```python
from build123d import *

# Parameters (mm, degrees)
F0_R     = 10.9728
F1_DEPTH = 6.9342


# Not quite as in the source:
# - a feature names something its author has since deleted; it is built from what else it names


with BuildPart() as f1:
    # F0 (on Front) → F1 (new body)
    with BuildSketch(Plane.XZ):
        with BuildLine():
            ThreePointArc((28.6439371533, 44.738406593), (31.7550616118, 42.5865732614), (34.7051660635, 40.2187967078))
            Line((34.7051660635, 40.2187967078), (38.3958422982, 44.2064153225))
            ThreePointArc((38.3958422982, 44.2064153225), (36.1509937048, 46.060324745), (33.8167671779, 47.8003568929))
            Line((33.8167671779, 47.8003568929), (28.6439371533, 44.738406593))
        make_face()
        with BuildLine():
            Line((38.3958422982, 44.2064153225), (34.7051660635, 40.2187967078))
            ThreePointArc((34.7051660635, 40.2187967078), (48.2991997583, 22.1175826623), (53.1225014483, 0))
            ThreePointArc((53.1225014483, 0), (24.8760182095, -46.9380855826), (-29.8247927528, -43.9600033823))
            Line((-29.8247927528, -43.9600033823), (-35.1168298869, -46.8535603786))
            ThreePointArc((-35.1168298869, -46.8535603786), (26.1940251259, -52.3671739658), (58.5529492123, 0))
            ThreePointArc((58.5529492123, 0), (53.2758747723, 24.2925714716), (38.3958422982, 44.2064153225))
        make_face()
        with BuildLine():
            ThreePointArc((33.8167671779, 47.8003568929), (36.1509937048, 46.060324745), (38.3958422982, 44.2064153225))
            Line((38.3958422982, 44.2064153225), (51.3007947444, 58.1496672696))
            Line((51.3007947444, 58.1496672696), (33.8167671779, 47.8003568929))
        make_face()
        with BuildLine():
            ThreePointArc((-37.1603482471, -37.9619372303), (-41.568846888, 33.0761413789), (28.6439371533, 44.738406593))
            Line((28.6439371533, 44.738406593), (33.8167671779, 47.8003568929))
            ThreePointArc((33.8167671779, 47.8003568929), (-44.9890332079, 37.475788884), (-40.9020715179, -41.898310312))
            Line((-40.9020715179, -41.898310312), (-37.1603482471, -37.9619372303))
        make_face()
        with BuildLine():
            Line((-35.1168298869, -46.8535603786), (-29.8247927528, -43.9600033823))
            ThreePointArc((-29.8247927528, -43.9600033823), (-33.6265739867, -41.1248547965), (-37.1603482471, -37.9619372303))
            Line((-37.1603482471, -37.9619372303), (-40.9020715179, -41.898310312))
            ThreePointArc((-40.9020715179, -41.898310312), (-38.090116415, -44.4701123559), (-35.1168298869, -46.8535603786))
        make_face()
        with BuildLine():
            Line((-56.9704473019, -58.8025860488), (-35.1168298869, -46.8535603786))
            ThreePointArc((-35.1168298869, -46.8535603786), (-38.090116415, -44.4701123559), (-40.9020715179, -41.898310312))
            Line((-40.9020715179, -41.898310312), (-56.9704473019, -58.8025860488))
        make_face()
        with BuildLine():
            Line((38.8165365087, 20.8673397533), (16.7947365087, 20.8673397533))
            Line((16.7947365087, 20.8673397533), (34.7051660635, 40.2187967078))
            ThreePointArc((34.7051660635, 40.2187967078), (31.7550616118, 42.5865732614), (28.6439371533, 44.738406593))
            Line((28.6439371533, 44.738406593), (-32.8515800228, 8.3374004968))
            Line((-32.8515800228, 8.3374004968), (-11.6390858311, 8.3374004968))
            Line((-11.6390858311, 8.3374004968), (-43.993112864, -21.982746443))
            Line((-43.993112864, -21.982746443), (-21.971312864, -21.982746443))
            Line((-21.971312864, -21.982746443), (-37.1603482471, -37.9619372303))
            ThreePointArc((-37.1603482471, -37.9619372303), (-33.6265739867, -41.1248547965), (-29.8247927528, -43.9600033823))
            Line((-29.8247927528, -43.9600033823), (31.308234758, -10.5339530787))
            Line((31.308234758, -10.5339530787), (10.099234758, -10.5339530787))
            Line((10.099234758, -10.5339530787), (38.8165365087, 20.8673397533))
        make_face()
        Circle(F0_R, mode=Mode.SUBTRACT)
    extrude(amount=F1_DEPTH)


solid = f1.part
```
CAD build for the part. Positions are in the model's coordinates, mm. A direction names the side the tool comes from. Round coordinates to 2 decimals unless told otherwise and drop trailing zeros. Loops run counter-clockwise (first coordinate to the right, second up) from the corner with the lowest first, then second, coordinate; pieces in that order, holes last. Notation, with made-up numbers: (89, 70.5) - (106, 70.5) arc R34 cw to (106, 107.5) - close; hole circle Ø3 at (36, 20). An arc over 180 degrees is marked (long way). Return JSON: item names as keys, results as strings. Group by question number.
Q1. Band-saw the part on B-B on z = -4.5. Give the cut face in (x, y).
Q2. Tool access for faces 1 (the face through (28, -3, 20.867)), 2 (the face through (42.681, -3.419, 53.047)), 3 (the face through (-46.197, -3.419, -52.912)), 4 (the face through (-1, -6.934, -12)): list every direction of +Z, -Z, +X, -X, +Y, -Y with a clear straight run to the whole face (end or side of a thin tool).
Q3. Drill centre lines: line 1 along Z through (x, y) = (1.5, -3.25); line 2 along Z through (x, y) = (-20, -2); line 3 along Z through (x, y) = (32.5, -5.5). Where is each one in solid material? Low to high. Write a range as [from, to].
Q4. Two-plate mould, pull along X, no slides. Class faces 5 (the face through (-48.82, -3.42, -50.23)), 6 (the face through (-1, 0, -12)), 7 (the face through (44.76, -3.42, 51.08)), 8 (the face through (-1.673, -3.419, 26.793)): +X half, -X half, draft (parallel to the pull), parting line (faces both ways), or undercut.
Q5. Band-saw the part on D-D on z = -40.5. Give the cut face in (x, y).
Q6. Band-saw the part on C-C on x = -15.5. Give the cut face in (y, z), plus the area to 3 significant figures.
Q7. Flat gauge pins, fed straight in: pin 1 Ø12 at (x, z) = (28.5, -21) entering from +Y; pin 2 Ø3 at (x, y) = (18, -4.5) entering from +Z; pin 3 Ø1.5 at (y, z) = (-2.5, -38.5) entering from -X; pin 4 Ø3.5 at (x, y) = (-19.5, -4.5) entering from -Z. Where does each tip first touch, or does it go through?
Solutions:
{
 "1": {"outline": "(-58.38, -6.93) - (-52.93, -6.93) - (-52.93, 0) - (-58.38, 0) - close; (-25.34, -6.93) - (-10.01, -6.93) - (-10.01, 0) - (-25.34, 0) - close; (10.01, -6.93) - (15.62, -6.93) - (15.62, 0) - (10.01, 0) - close; (52.93, -6.93) - (58.38, -6.93) - (58.38, 0) - (52.93, 0) - close"},
 "2": {"face 1": "+Y, -Y", "face 2": "+Z, +Y, -Y", "face 3": "-Z, +Y, -Y", "face 4": "+Z, -Z, +X, -X, -Y"},
 "3": {"line 1": "z = [-58.53, -53.1], [-26.83, -10.87], [10.87, 28.67], [53.1, 58.53]", "line 2": "z = [-55.03, -49.21], [-38.59, 0.5], [8.34, 15.94], [49.21, 55.03]", "line 3": "z = [-48.71, -42.02], [13.96, 20.87], [37.84, 48.71]"},
 "4": {"face 5": "-X half", "face 6": "draft", "face 7": "+X half", "face 8": "undercut"},
 "5": {"outline": "(-42.29, -6.93) - (-23.5, -6.93) - (-23.5, 0) - (-42.29, 0) - close; (34.38, -6.93) - (42.29, -6.93) - (42.29, 0) - (34.38, 0) - close"},
 "6": {"outline": "(-6.93, -56.46) - (0, -56.46) - (0, -50.81) - (-6.93, -50.81) - close; (-6.93, -36.13) - (0, -36.13) - (0, 4.72) - (-6.93, 4.72) - close; (-6.93, 8.34) - (0, 8.34) - (0, 18.61) - (-6.93, 18.61) - close; (-6.93, 50.81) - (0, 50.81) - (0, 56.46) - (-6.93, 56.46) - close", "area": "433 mm^2"},
 "7": {"pin 1": "passes through", "pin 2": "stops at z = 56.18", "pin 3": "stops at x = -44.76", "pin 4": "stops at z = -55.8"}
}
